from build123d import *

# Parameters (mm, degrees)
RESSALTO_EXTRUS_O1_DEPTH = 5
ESBO_O2_W                = 95
ESBO_O2_H                = 5
RESSALTO_EXTRUS_O2_DEPTH = 5
ESBO_O5_W                = 5
ESBO_O5_H                = 2
CORTE_EXTRUS_O1_DEPTH    = 10
CORTE_EXTRUS_O2_DEPTH    = 10
ESBO_O8_R                = 3.075
CORTE_EXTRUS_O3_DEPTH    = 6
CORTE_EXTRUS_O4_DEPTH    = 10
ESBO_O10_R               = 1.5
CORTE_EXTRUS_O5_DEPTH    = 10


with BuildPart() as part:
    # Esboço1 → Ressalto-extrusão1 (new body)
    with BuildSketch(Plane.XY):
        Polygon((-44.712278576, -7.96460177), (-24.712278576, 12.03539823), (55.287721424, 12.03539823), (55.287721424, -7.96460177), align=None)
    extrude(amount=RESSALTO_EXTRUS_O1_DEPTH)

    # Esboço2 → Ressalto-extrusão2 (add)
    with BuildSketch(Plane.XZ.offset(7.96460177)):
        with Locations((2.787721424, 2.5)):
            Rectangle(ESBO_O2_W, ESBO_O2_H)
    extrude(amount=RESSALTO_EXTRUS_O2_DEPTH)

    # Esboço5 → Corte-extrusão1 (cut)
    with BuildSketch(Plane(origin=(-18.373838403, 18.373838403, 0), x_dir=(0, 0, 1), z_dir=(-0.707106781, 0.707106781, 0))):
        with Locations((2.5, -14.963908057)):
            Rectangle(ESBO_O5_W, ESBO_O5_H)
    extrude(amount=-CORTE_EXTRUS_O1_DEPTH, mode=Mode.SUBTRACT)

    # Esboço7 → Corte-extrusão2 (cut)
    with BuildSketch(Plane.XY.offset(5)):
        Polygon((-24.712278576, 4.964330418), (-23.460699574, 6.215909421), (-21.72828796, 4.483497807), (-22.979866962, 3.231918804), align=None)
        Polygon((-24.394080525, 1.817705242), (-25.645659528, 0.566126239), (-27.378071141, 2.298537853), (-26.126492139, 3.550116856), align=None)
    extrude(amount=-CORTE_EXTRUS_O2_DEPTH, mode=Mode.SUBTRACT)

    # Esboço8 → Corte-extrusão3 (cut, through all)
    with BuildSketch(Plane.XY.offset(5)):
        with Locations((-4.712278576, -0.46460177)):
            Circle(ESBO_O8_R)
    extrude(amount=-CORTE_EXTRUS_O3_DEPTH, mode=Mode.SUBTRACT)

    # Esboço9 → Corte-extrusão4 (cut)
    with BuildSketch(Plane.XY.offset(5)):
        with BuildLine():
            Line((12.777721424, 7.03539823), (42.797721424, 7.03539823))
            ThreePointArc((42.797721424, 7.03539823), (44.558417309, 6.306094115), (45.287721424, 4.54539823))
            Line((45.287721424, 4.54539823), (45.287721424, 4.52539823))
            ThreePointArc((45.287721424, 4.52539823), (44.558417309, 2.764702345), (42.797721424, 2.03539823))
            Line((42.797721424, 2.03539823), (12.777721424, 2.03539823))
            ThreePointArc((12.777721424, 2.03539823), (11.017025538, 2.764702345), (10.287721424, 4.52539823))
            Line((10.287721424, 4.52539823), (10.287721424, 4.54539823))
            ThreePointArc((10.287721424, 4.54539823), (11.017025538, 6.306094115), (12.777721424, 7.03539823))
        make_face()
        with BuildLine():
            Line((12.777721424, -2.96460177), (42.797721424, -2.96460177))
            ThreePointArc((42.797721424, -2.96460177), (44.558417309, -3.693905885), (45.287721424, -5.45460177))
            Line((45.287721424, -5.45460177), (45.287721424, -5.47460177))
            ThreePointArc((45.287721424, -5.47460177), (44.558417309, -7.235297655), (42.797721424, -7.96460177))
            Line((42.797721424, -7.96460177), (12.777721424, -7.96460177))
            ThreePointArc((12.777721424, -7.96460177), (11.017025538, -7.235297655), (10.287721424, -5.47460177))
            Line((10.287721424, -5.47460177), (10.287721424, -5.45460177))
            ThreePointArc((10.287721424, -5.45460177), (11.017025538, -3.693905885), (12.777721424, -2.96460177))
        make_face()
    extrude(amount=-CORTE_EXTRUS_O4_DEPTH, mode=Mode.SUBTRACT)

    # Esboço10 → Corte-extrusão5 (cut)
    with BuildSketch(Plane.XY.offset(5)):
        with Locations((52.787721424, 7.03539823)):
            Circle(ESBO_O10_R)
        with Locations((52.787721424, -2.96460177)):
            Circle(ESBO_O10_R)
    extrude(amount=-CORTE_EXTRUS_O5_DEPTH, mode=Mode.SUBTRACT)


solid = part.part
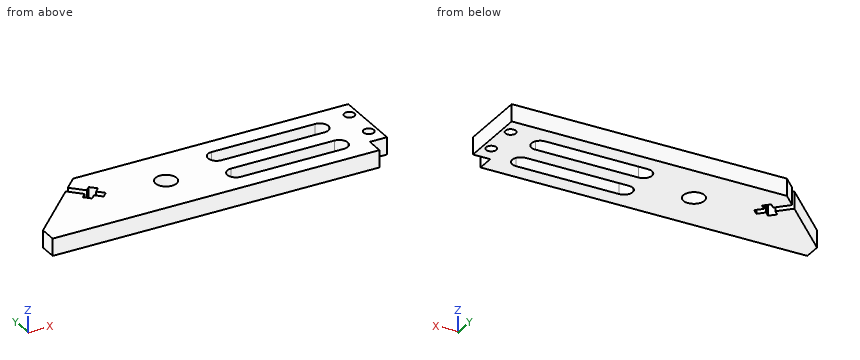
Part model, mm, in its own coordinate system. Coordinates: 2 decimals unless noted, no trailing zeros. Loops run counter-clockwise (first coordinate to the right, second up) from the corner with the lowest first, then second, coordinate; pieces in that order, holes last. Notation, with made-up numbers: (63.5, 29.25) - (101.5, 29.25) arc R14 cw to (101.5, 51.25) - close; hole circle Ø2 at (69, 24). An arc over 180 degrees is marked (long way). Write each question's results on one line, items separated by ' | '. Start each with the question number.
Q1. Slice it at A-A on x = 16.5. Give the cut face in (y, z), and give its area (3 significant figures).
Q2. Probe line 1 along Y through (x, z) = (15.5, 1.9); line 2 along X through (y, z) = (1, 3.8); line 3 along Y through (x, z) = (12, 1.4). List the from-to ranges inside material, lowest first.
Q3. Drop flat-ended pins along their axis: pin 1 Ø2 at (y, z) = (8.5, 2) entering from -X; pin 2 Ø2.5 at (x, y) = (52.79, 7.04) entering from +Z. Give the stop position or say it passes through.
Q4. Slice it at C-C on z = 3.75. Give the number of separate pieces and of enclosed holes in the cut face, and give its area (3 significant figures).
Q5. Slice it at B-B on y = -10.5. Give the cut face in (x, z), and give its area (3 significant figures).
Answer:
1) outline: (-12.96, 0) - (-7.96, 0) - (-7.96, 5) - (-12.96, 5) - close; (-2.96, 0) - (2.04, 0) - (2.04, 5) - (-2.96, 5) - close; (7.04, 0) - (12.04, 0) - (12.04, 5) - (7.04, 5) - close | area: 75.0 mm2
2) line 1: y = -12.96 to -7.96, -2.96 to 2.04, 7.04 to 12.04 | line 2: x = -35.75 to -26.08, -25.21 to -23.58, -21.61 to -7.42, -2.01 to 55.29 | line 3: y = -12.96 to -7.84, -3.09 to 2.16, 6.91 to 12.04
3) pin 1: stops at x = -28.25 | pin 2: passes through
4) separate pieces: 1 | enclosed holes: 5 | area: 1,860 mm2
5) outline: (-44.71, 0) - (50.29, 0) - (50.29, 5) - (-44.71, 5) - close | area: 475 mm2
